Autodesk Inventor part; units mm, degrees
ref_plane "YZ Plane" through (0, 0, 0) normal (1, 0, 0) x (0, 1, 0)
ref_plane "XZ Plane" through (0, 0, 0) normal (0, 1, 0) x (-1, 0, 0)
ref_plane "XY Plane" through (0, 0, 0) normal (0, 0, 1) x (1, 0, 0)
sketch "Boceto1" plane through (0, 0, 0) normal (0, 1, 0) x (-1, 0, 0)
  line L0 (-12.5, -30) -> (12.5, -30)
  line L1 (12.5, -30) -> (12.5, 30)
  line L2 (12.5, 30) -> (-12.5, 30)
  line L3 (-12.5, 30) -> (-12.5, -30)
  line L4 (-12.5, -30) -> (12.5, 30) construction
  line L5 (12.5, -30) -> (-12.5, 30) construction
  line L6 (61.5, -13) -> (11.5, -13)
  line L7 (11.5, -13) -> (11.5, 13)
  line L8 (11.5, 13) -> (61.5, 13)
  line L9 (61.5, 13) -> (61.5, -13)
  line L10 (12.5, 0) -> (11.5, 0) construction
  point P0 (0, 0)
  point P1 (12.5, 13)
  point P2 (12.5, -13)
  dimension "d0" = 25
  dimension "d1" = 60
  dimension "d8" = 50
  dimension "d9" = 26
  dimension "d10" = 1
extrude "Extrusión1" add sketch "Boceto1" along normal blind 5 contours L3 L2 L1 L8 L7 L6 L0 | L6 L7 L8 L1
sketch "Boceto2" plane through (-12.5, 0, 30) normal (0, 0, 1) x (1, 0, 0)
  circle A0 centre (-3.9208, 2.5) radius 1.65
  line L0 (0, 0) -> (0, 5) construction
  line L1 (0, 2.5) -> (-8.4797, 2.5) construction
  circle A1 centre (-3.9208, 2.5) radius 4.65
  line L2 (-2.2708, 2.5) -> (0, 0)
  line L3 (-2.2708, 2.5) -> (-26.7468, 29.4468) construction
  line L4 (-6.0334, 6.6424) -> (-3.6387, -2.1414)
  line L5 (0, 5) -> (25, 5)
  line L6 (-3.7417, 7.1465) -> (25, 7.1465)
  line L7 (25, 7.1465) -> (25, 5)
  line L8 (25, 5) -> (-3.7417, 5)
  line L9 (-3.7417, 5) -> (-3.7417, 7.1465)
  arc A2 (0, 0) -> (0.7292, 2.5) centre (-3.9208, 2.5) ccw
  line L10 (-6.0334, 6.6424) -> (-1.5623, -1.5075) construction
  point P0 (12.5, 0)
  point P1 (-4.481, 0.948)
  dimension "d4" = 3.3
  dimension "d5" = 3
extrude "Extrusión2" add sketch "Boceto2" against normal blind 60 contours A0 L4 A1 L9 L8 L2 | A0 L4 A1 | L6 L7 L5 A1 | A1 L8 L9
extrude "Extrusión3" cut sketch "Boceto1" along normal through all both and the other way through all contours L6 L7 L8 L1 | L1 L8 L9 L6
sketch "Boceto3" plane through (-16.2417, 7.1465, 30) normal (0, 0, 1) x (1, 0, 0)
  line L0 (3.7417, -7.1465) -> (28.7417, -7.1465)
  line L1 (28.7417, -7.1465) -> (28.7417, 0)
  line L2 (3.7417, -7.1465) -> (28.7417, -7.1465)
  line L3 (28.7417, -7.1465) -> (28.7417, -4.1465)
  line L4 (28.7417, -4.1465) -> (3.7417, -4.1465)
  line L5 (3.7417, -4.1465) -> (3.7417, -7.1465)
  line L6 (3.7417, -7.1465) -> (6.7417, -4.1465)
  line L7 (3.7417, -7.1465) -> (7.9843, -7.1465) construction
  point P0 (16.2417, -7.1465)
  dimension "d13" = 3
  dimension "d16" = 45
extrude "Extrusión4" cut sketch "Boceto3" against normal blind 60 contours L6 L4 L1 L0
extrude "Extrusión5" cut sketch "Boceto3" along normal up to surface (26 mm away) from surface at -43 contours L5 L4 L6
fillet "Empalme1" radius 2 2 edges at (12.5, 7.1465, 0) (12.5, 3, 0)
fillet "Empalme2" radius 2 10 edges at (11.9142, 6.5608, 30) (12.5, 5.0733, 30) (11.9142, 3.5858, 30) (0.5, 3, 30) (-2.8708, 7.1465, 30) (11.9142, 6.5608, -30) (12.5, 5.0733, -30) (11.9142, 3.5858, -30) (0.5, 3, -30) (-2.8708, 7.1465, -30)
Source: CAD feature listing. Evaluate the final solid. Frame: model axes, mm. A direction names the side the tool comes from. Round coordinates to 2 decimals unless told otherwise and drop trailing zeros. Write each loop counter-clockwise with the first axis right and the second up, starting at its lowest first coordinate (ties: lowest second). Pieces come first, ordered by that corner, then holes. Notation, with made-up numbers: M 33,59 L 53,59 A36 ccw 53,93 Z; hole C 27.5,-4 d5. An arc over 180 degrees is marked long. Answer as a JSON object with one key per item and string values. Group by question number.
(1) Section query C-C on x = -15.5. Output: boundary loops of the cut face in (y, z).
(2) Section query D-D on z = 17.5. Output: boundary loops of the cut face in (x, y), then the cut area to 3 significant figures.
(3) First-contact query: pin 1 (4 mm diameter, centred on x = 8, y = 2, fed in from -Z); pin 2 (2 mm diameter, centred on y = 5.5, z = 18, fed in from -X); pin 3 (1.2 mm diameter, centred on y = 4.5, z = -4.5, fed in from -X). Flat tips, straight axial feed; report the tip coordinate or a pass-through.
(4) Section query B-B on z = 7. Output: boundary loops of the cut face in (x, y), then the cut area to 3 significant figures.
(5) Mould query, pull axis Z, two halves, no side actions, for faces 1 (the cylindrical face through (11.899, 6.576, -0.392)), 2 (the flat face through (-15, 5, -13)), 3 (the cylindrical face through (0.64, 3.6, 29.43)). Classes: +Z half, -Z half, draft (parallel to the pull), parting line (faces both ways), or undercut.
(6) Ray query, line 1 (X direction, y = 2.5, z = 24.5); line 2 (Y direction, x = 10.5, z = -3.5); line 3 (Y direction, x = -11.5, z = -20). Return the intervals inside material, ascending. Write a range as [from, to].
(7) Reachability of faces 4 (the cylindrical face through (0.64, 3.57, -29.4)), 5 (the flat face through (-16.566, -0.575, 21.619)), 6 (the cylindrical face through (-3.057, 6.545, 29.43)) from +Z, -Z, +X, -X, +Y, -Y: full face, straight path, thin tool, end or side. Return the list, or none.
(8) Section query A-A on x = -4.5. Output: boundary loops of the cut face in (y, z).
Computed values:
{
 "1": {"outline": "M 3.87,-30 L 7.06,-30 L 7.06,-28.59 A2 ccw 7.15,-28 L 7.15,-13 L 3.87,-13 Z; M 3.87,13 L 7.15,13 L 7.15,28 A2 ccw 7.06,28.59 L 7.06,30 L 3.87,30 Z"},
 "2": {"outline": "M -16.98,0.95 A1.65 cw long -14.77,2.5 L -12.5,0 L -9.5,3 L 10.5,3 A2 ccw 12.5,5 L 12.5,5.15 A2 ccw 10.5,7.15 L -16.24,7.15 A4.65 ccw long -16.14,-2.14 Z", "area": "155 mm^2"},
 "3": {"pin 1": "z = -29.73", "pin 2": "x = -20.62", "pin 3": "x = -11.5"},
 "4": {"outline": "M -11.5,3 L 10.5,3 A2 ccw 12.5,5 L 12.5,5.15 A2 ccw 10.5,7.15 L -11.5,7.15 Z", "area": "97.8 mm^2"},
 "5": {"face 1": "draft", "face 2": "undercut", "face 3": "+Z half"},
 "6": {"line 1": "[-21.07, -18.07], [-14.77, -10]", "line 2": "[3, 7.15]", "line 3": "[1, 7.15]"},
 "7": {"face 4": "-Z, +X, -Y", "face 5": "+Z, -Z", "face 6": "+Z, +X, +Y"},
 "8": {"outline": "M 3,-28 A2 ccw 5,-30 L 5.15,-30 A2 ccw 7.15,-28 L 7.15,28 A2 ccw 5.15,30 L 5,30 A2 ccw 3,28 Z"}
}
